Build history of the part. All positions in model axes, mm. A direction names the side the tool comes from. Round coordinates to 2 decimals unless told otherwise and drop trailing zeros. Loops run counter-clockwise (first coordinate to the right, second up) from the corner with the lowest first, then second, coordinate; pieces in that order, holes last. Notation, with made-up numbers: (40, -3) - (90, -3) arc R24 ccw to (90, 24) - close; hole circle Ø4 at (54, -23.5). An arc over 180 degrees is marked (long way). Use a Markdown table: item, result.
from build123d import *

# Parameters (mm, degrees)
SKETCH1_R           = 3
BOSS_EXTRUDE1_DEPTH = 5
SKETCH2_R           = 10
BOSS_EXTRUDE2_DEPTH = 3
SKETCH3_R           = 1.4
CUT_EXTRUDE1_DEPTH  = 3
CIRPATTERN1_COUNT   = 3
CHAMFER1_SIZE       = 1


with BuildPart() as part:
    # Sketch1 → Boss-Extrude1 (new body)
    with BuildSketch(Plane.XY):
        Circle(SKETCH1_R)
    extrude(amount=BOSS_EXTRUDE1_DEPTH)

    # Sketch2 → Boss-Extrude2 (add)
    with BuildSketch(Plane.XY.offset(5)):
        Circle(SKETCH2_R)
    extrude(amount=BOSS_EXTRUDE2_DEPTH)

    # Sketch3 → Cut-Extrude1 (cut)
    with BuildSketch(Plane.XY.offset(8)):
        with Locations((0, 6)):
            Circle(SKETCH3_R)
    cut_extrude1 = extrude(amount=-CUT_EXTRUDE1_DEPTH, mode=Mode.SUBTRACT)

    # CirPattern1: Cut-Extrude1 ×3 about axis
    cirpattern1_axis = Axis((0, 0, 0), (0, 0, 1))
    for i in range(1, CIRPATTERN1_COUNT):
        add(cut_extrude1.rotate(cirpattern1_axis, i * 360 / CIRPATTERN1_COUNT), mode=Mode.SUBTRACT)

    # Chamfer1
    chamfer1_edges = [part.edges().sort_by_distance(p)[0] for p in [
        (-3, 0, 0),
    ]]
    chamfer(chamfer1_edges, length=CHAMFER1_SIZE)


solid = part.part
Q1. Cut at A-A, the plane x = 0. List the corners of the cut face in (y, z).
Results found:
| item | result |
|---|---|
| outline | (-10, 5) - (-3, 5) - (-3, 1) - (-2, 0) - (2, 0) - (3, 1) - (3, 5) - (4.6, 5) - (4.6, 8) - (-10, 8) - close; (7.4, 5) - (10, 5) - (10, 8) - (7.4, 8) - close |
Q2. Cut at C-C, the plane y = 0. List the corners of the cut face in (x, z).
Results found:
| item | result |
|---|---|
| outline | (-10, 5) - (-3, 5) - (-3, 1) - (-2, 0) - (2, 0) - (3, 1) - (3, 5) - (10, 5) - (10, 8) - (-10, 8) - close |
Q3. Probe line 1 (Z direction, x = 7.25, y = 6.75); line 2 (Y direction, x = -6.25, z = 7.75); line 3 (Y direction, x = 5.5, z = 7.25). List the from-to ranges inside material, lowest first.
Results found:
| item | result |
|---|---|
| line 1 | z = 5 to 8 |
| line 2 | y = -7.81 to -3.92, -2.08 to 7.81 |
| line 3 | y = -8.35 to -4.37, -1.63 to 8.35 |
Q4. Which spindle directions (+Z, -Z, +X, -X, +Y, -Y) get a long thin tool onto all of the face, cutting with end or side? Do faces 4 (the face through (3.8, -2.9, 6.5)), 5 (the face through (-3, 0, 3)). Say none if no direction does.
Results found:
| item | result |
|---|---|
| face 4 | +Z, -Z |
| face 5 | -Z |
Q5. Pull direction Y, two halves, no side cores. Call faces 1 (the face through (-0.18, 7.39, 6.52)), 2 (the face through (0, 0, 0)), 3 (the face through (-2.17, -9.76, 6.48)): pulls with the +Y half, pulls with the -Y half, needs draft (parallel to the pull), parting line crosses it, or undercut.
Results found:
| item | result |
|---|---|
| face 1 | undercut |
| face 2 | needs draft |
| face 3 | parting line crosses it |
Q6. Cut at D-D, the plane z = 3.75. List the corners of the cut face in (x, y).
Results found:
| item | result |
|---|---|
| outline | circle Ø6 at (0, 0) |
Q7. Drop flat-ended pins along their axis: pin 1 (2.5 mm diameter, centred on x = 5.2, y = -3, fed in from +Z); pin 2 (1.5 mm diameter, centred on x = 2.5, z = 3, fed in from +Y); pin 3 (3.5 mm diameter, centred on x = -5.2, y = -3, fed in from -Z). Give the stop position or say it passes through.
Results found:
| item | result |
|---|---|
| pin 1 | passes through |
| pin 2 | stops at y = 2.44 |
| pin 3 | stops at z = 5 |
Q8. Cut at B-B, the plane y = 6. List the corners of the cut face in (x, z), plus the area to 3 significant figures.
Results found:
| item | result |
|---|---|
| outline | (-8, 5) - (-1.4, 5) - (-1.4, 8) - (-8, 8) - close; (1.4, 5) - (8, 5) - (8, 8) - (1.4, 8) - close |
| area | 39.6 mm2 |
